Could you check a few things on this model? Use its own coordinates, in mm. Face numbers are marked on the shaded views. A direction names the side the tool comes from. Round coordinates to 2 decimals unless told otherwise and drop trailing zeros. Loops run counter-clockwise (first coordinate to the right, second up) from the corner with the lowest first, then second, coordinate; pieces in that order, holes last. Notation, with made-up numbers: M 58,65 L 93,65 A35 cw 93,98 Z; hole C -28.75,-39 d2. An arc over 180 degrees is marked long. One line per item, written item: value. Start each with the question number.
Q1. Imagine slicing it at D-D (z = 16). Please give me the cut outline in (x, y), then the cut area to 3 significant figures.
Q2. Imagine slicing it at B-B (x = -45). Please give me the cut outline in (y, z).
Q3. Imagine slicing it at C-C (y = 98.5). Please give me the cut outline in (x, z), then the cut area to 3 significant figures.
Q4. Imagine slicing it at A-A (z = 45). Please give me the cut outline in (x, y).
Q5. Please list where these lines run through material, in increasing order: line 1 along X through (y, z) = (154, -45); line 2 along Y through (x, z) = (-21, 43); line 3 along Z through (x, y) = (-4.5, 14).
Q6. I'm going to push flat-ended pins straight in: pin 1 Ø12 at (y, z) = (47.5, -8) entering from +X; pin 2 Ø1.5 at (x, z) = (31.5, 7) entering from -Y; pin 3 Ø3 at (y, z) = (96.5, -5) entering from -X; pin 4 Ø24 at (x, z) = (45, -45) entering from +Y. Where does each tip first touch, or does it pass through?
Q7. Which directions (+Z, -Z, +X, -X, +Y, -Y) give clear straight access to the entire face, cutting with the end or side of a thin tool? Please do the marked faces 1, 2, 3 and 4.
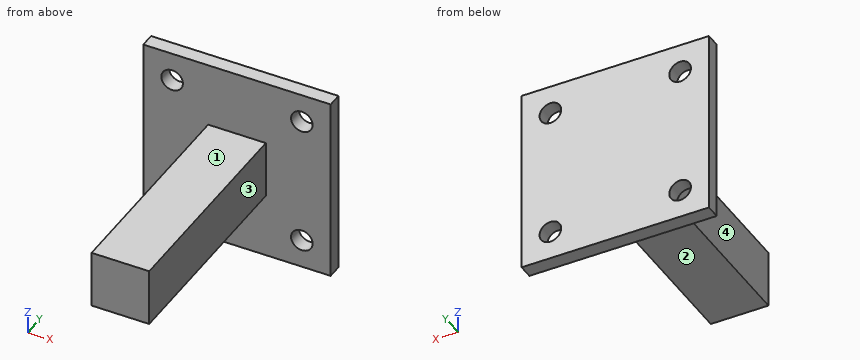
from build123d import *

# Parameters (mm, degrees)
SKETCH1_W           = 40
SKETCH1_H           = 40
BOSS_EXTRUDE1_DEPTH = 150
SKETCH2_W           = 130
SKETCH2_H           = 130
SKETCH2_R           = 7.5
BOSS_EXTRUDE2_DEPTH = 10


with BuildPart() as part:
    # Sketch1 → Boss-Extrude1 (new body)
    with BuildSketch(Plane(origin=(0, 0, 0), x_dir=(1, 0, 0), z_dir=(0, 1, 0))):
        Rectangle(SKETCH1_W, SKETCH1_H)
    extrude(amount=BOSS_EXTRUDE1_DEPTH)

    # Sketch2 → Boss-Extrude2 (add)
    with BuildSketch(Plane(origin=(0, 150, 0), x_dir=(1, 0, 0), z_dir=(0, 1, 0))):
        Rectangle(SKETCH2_W, SKETCH2_H)
        with Locations(Location((-45, -45, 0), (0, 0, 270))):
            Circle(SKETCH2_R, mode=Mode.SUBTRACT)
        with Locations(Location((45, -45, 0), (0, 0, 270))):
            Circle(SKETCH2_R, mode=Mode.SUBTRACT)
        with Locations(Location((45, 45, 0), (0, 0, 270))):
            Circle(SKETCH2_R, mode=Mode.SUBTRACT)
        with Locations(Location((-45, 45, 0), (0, 0, 270))):
            Circle(SKETCH2_R, mode=Mode.SUBTRACT)
    extrude(amount=BOSS_EXTRUDE2_DEPTH)


solid = part.part
Report:
1. outline: M -65,150 L -20,150 L -20,0 L 20,0 L 20,150 L 65,150 L 65,160 L -65,160 Z
1. area: 7,300 mm²
2. outline: M 150,-65 L 160,-65 L 160,-52.5 L 150,-52.5 Z; M 150,-37.5 L 160,-37.5 L 160,37.5 L 150,37.5 Z; M 150,52.5 L 160,52.5 L 160,65 L 150,65 Z
3. outline: M -20,-20 L 20,-20 L 20,20 L -20,20 Z
3. area: 1,600 mm²
4. outline: M -65,150 L -52.5,150 L -52.5,160 L -65,160 Z; M -37.5,150 L 37.5,150 L 37.5,160 L -37.5,160 Z; M 52.5,150 L 65,150 L 65,160 L 52.5,160 Z
5. line 1: x = -65 to -52.5, -37.5 to 37.5, 52.5 to 65
5. line 2: y = 150 to 160
5. line 3: z = -20 to 20
6. pin 1: stops at x = 20
6. pin 2: stops at y = 150
6. pin 3: stops at x = -20
6. pin 4: stops at y = 160
7. face 1: +Z, +X, -X, -Y
7. face 2: -Z, +X, -X, -Y
7. face 3: +Z, -Z, +X, -Y
7. face 4: +Z, -Z, -X, -Y
